Could you check a few things on this model? Use its own coordinates, in mm. Face numbers are marked on the shaded views. A direction names the side the tool comes from. Round coordinates to 2 decimals unless told otherwise and drop trailing zeros. Loops run counter-clockwise (first coordinate to the right, second up) from the corner with the lowest first, then second, coordinate; pieces in that order, holes last. Notation, with made-up numbers: (15.25, 20) -> (71.25, 20) arc R15 cw to (71.25, 29) -> close; hole circle Ø6 at (-29.75, 49). An arc over 180 degrees is marked (long way). Put each result on its own line as item: value. Start each with the question number.
1. I'm going to push flat-ended pins straight in: P1, Ø5, axis at y = 20, z = 40, coming from the +X side; P2, Ø10, axis at y = -9.5, z = 64, coming from the -X side; P3, Ø12, axis at y = -9, z = 107, coming from the +X side; P4, Ø4, axis at x = -3.5, y = -0.5, coming from the -Z side. Where does each tip first touch, or does it pass through?
2. Imagine slicing it at A-A, the plane x = 0. Please give me the cut outline in (y, z), and give its area (3 significant figures).
3. Imagine slicing it at D-D, the plane z = 146.5. Please give me the cut outline in (x, y), and give its area (3 significant figures).
4. I need wall thicknesses on line 1 (Z direction, x = -10, y = 18.5); line 2 (Z direction, x = 1, y = 17.5); line 3 (Y direction, x = 1, z = 61). Which ranges of each line are inside material? Lowest first, please. Write a range as [from, to].
5. Imagine slicing it at B-B, the plane y = 19. Please give me the cut outline in (x, z).
6. Which directions (+Z, -Z, +X, -X, +Y, -Y) give clear straight access to the entire face, cutting with the end or side of a thin tool? Please do the marked faces 1, 2 and 3.
7. Imagine slicing it at C-C, the plane y = -17.5. Please give me the cut outline in (x, z), and give its area (3 significant figures).
8. If we mould it in two halves opening along Z, with no side actions, what happens to the marked faces 4, 5 and 6? For each: pulls with the +Z half, pulls with the -Z half, needs draft (parallel to the pull), parting line crosses it, or undercut.
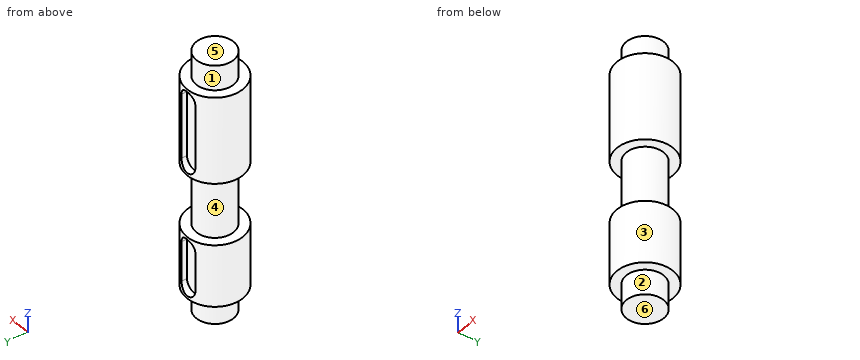
Autodesk Inventor part; units mm, degrees
sketch "スケッチ1" plane through (0, 0, 0) normal (0, 0, 1) x (1, 0, 0)
  point P0 (0, 0)
ref_plane "作業平面1" through (0, 0, 45) normal (0, 0, 1) x (1, 0, 0)
ref_plane "作業平面2" through (0, 0, 155) normal (0, 0, 1) x (1, 0, 0)
ref_plane "作業平面3" through (0, 0, 210) normal (0, 0, 1) x (1, 0, 0)
sketch "スケッチ2" plane through (0, 0, 45) normal (0, 0, 1) x (1, 0, 0)
  circle A0 centre (0, 0) radius 22.5
  dimension "d3" = 45
extrude "押し出し1" add sketch "スケッチ2" along normal blind 25
sketch "スケッチ3" plane through (0, 0, 155) normal (0, 0, 1) x (1, 0, 0)
  circle A0 centre (0, 0) radius 22.5
  dimension "d6" = 45
extrude "押し出し2" add sketch "スケッチ3" along normal blind 35
ref_plane "作業平面5" through (0, 22.5, 0) normal (0, 1, 0) x (-1, 0, 0)
sketch "スケッチ5" plane through (0, 22.5, 0) normal (0, 1, 0) x (-1, 0, 0)
  line L0 (22.5, 45) -> (-22.5, 45)
  line L1 (0, 45) -> (0, 65)
  line L2 (0, 65) -> (0, 61)
  arc A0 (7, 61) -> (-7, 61) centre (0, 61) ccw
  line L3 (7, 61) -> (7, 45)
  line L4 (7, 45) -> (-7, 45)
  line L5 (-7, 61) -> (-7, 45)
  line L6 (7, 45) -> (-7, 45)
  point P0 (0, 0)
  point P1 (-4, 61)
  dimension "d11" = 20
  dimension "d12" = 4
  dimension "d13" = 7
extrude "押し出し3" cut sketch "スケッチ5" against normal blind 5.5
mirror "ミラー1" about plane through (0, 0, 45) normal (0, 0, 1) of "押し出し1", "押し出し3"
sketch "スケッチ6" plane through (0, 22.5, 0) normal (0, 1, 0) x (-1, 0, 0)
  line L0 (22.5, 155) -> (-22.5, 155)
  line L1 (0, 155) -> (0, 185)
  line L2 (0, 185) -> (0, 181)
  arc A0 (7, 181) -> (-7, 181) centre (0, 181) ccw
  line L3 (7, 181) -> (7, 155)
  line L4 (-7, 155) -> (-7, 181)
  line L5 (7, 155) -> (-7, 155)
  point P0 (0, 0)
  dimension "d16" = 30
  dimension "d17" = 4
  dimension "d18" = 7
extrude "押し出し4" cut sketch "スケッチ6" against normal blind 5.5
mirror "ミラー2" about plane through (0, 0, 155) normal (0, 0, -1) of "押し出し4", "押し出し2"
sketch "スケッチ7" plane through (0, 0, 0) normal (0, 0, 1) x (1, 0, 0)
  circle A0 centre (0, 0) radius 15
  dimension "d21" = 30
extrude "押し出し5" add sketch "スケッチ7" along normal blind 210
properties part number "shift2"
Entries:
1. P1: x = 14.14
1. P2: x = -22.05
1. P3: x = 14.7
1. P4: z = 0
2. outline: (-22.5, 20) -> (-15, 20) -> (-15, 0) -> (15, 0) -> (15, 20) -> (22.5, 20) -> (22.5, 22) -> (17, 22) -> (17, 68) -> (22.5, 68) -> (22.5, 70) -> (15, 70) -> (15, 120) -> (22.5, 120) -> (22.5, 122) -> (17, 122) -> (17, 188) -> (22.5, 188) -> (22.5, 190) -> (15, 190) -> (15, 210) -> (-15, 210) -> (-15, 190) -> (-22.5, 190) -> (-22.5, 120) -> (-15, 120) -> (-15, 70) -> (-22.5, 70) -> close
2. area: 7,480 mm^2
3. outline: (-7, 17) -> (-7, 21.38) arc R22.5 ccw (long way) to (7, 21.38) -> (7, 17) -> close
3. area: 1,520 mm^2
4. line 1: [20, 70], [120, 190]
4. line 2: [20, 22.07], [67.93, 70], [120, 122.07], [187.93, 190]
4. line 3: [-22.48, 17]
5. outline: (-12.05, 20) -> (12.05, 20) -> (12.05, 70) -> (-12.05, 70) -> close; (-12.05, 120) -> (12.05, 120) -> (12.05, 190) -> (-12.05, 190) -> close; hole (-7, 29) arc R7 ccw to (7, 29) -> (7, 61) arc R7 ccw to (-7, 61) -> close; hole (-7, 129) arc R7 ccw to (7, 129) -> (7, 181) arc R7 ccw to (-7, 181) -> close
6. face 1: +Z
6. face 2: -Z
6. face 3: +Z, -Z
7. outline: (-14.14, 20) -> (14.14, 20) -> (14.14, 70) -> (-14.14, 70) -> close; (-14.14, 120) -> (14.14, 120) -> (14.14, 190) -> (-14.14, 190) -> close
7. area: 3,390 mm^2
8. face 4: undercut
8. face 5: pulls with the +Z half
8. face 6: pulls with the -Z half
